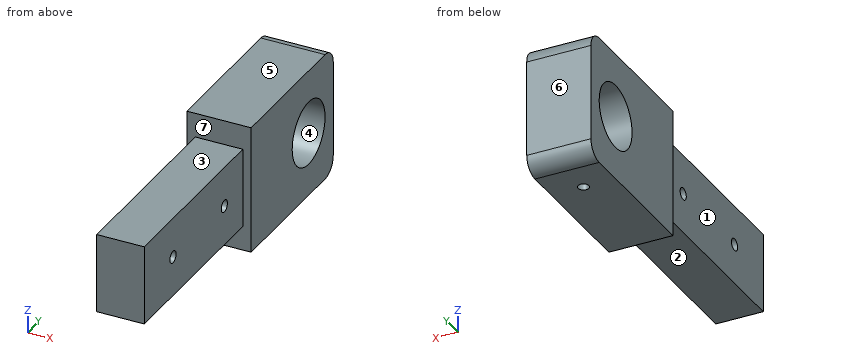
```python
from build123d import *

# Parameters (mm, degrees)
SKETCH2_W               = 20.828
SKETCH2_H               = 33.528
BOSS_EXTRUDE1_DEPTH     = 76.2
SKETCH3_W               = 25.4
SKETCH3_H               = 50.8
BOSS_EXTRUDE2_DEPTH     = 63.5
FILLET1_R               = 6.35
SKETCH4_R               = 12.7
CUT_EXTRUDE1_DEPTH      = 145.244271983
CUT_EXTRUDE2_REACH      = 151.191
CUT_EXTRUDE2_END_RADIUS = 12.7
SKETCH5_R               = 2.15265
SKETCH6_W               = 20.828
SKETCH6_H               = 33.528
CUT_EXTRUDE3_DEPTH      = 76.2
SKETCH7_R               = 2.38125
CUT_EXTRUDE4_DEPTH      = 78.74


with BuildPart() as part:
    # Sketch2 → Boss-Extrude1 (new body)
    with BuildSketch(Plane(origin=(0, 0, 0), x_dir=(1, 0, 0), z_dir=(0, 1, 0))):
        Rectangle(SKETCH2_W, SKETCH2_H)
    extrude(amount=BOSS_EXTRUDE1_DEPTH)

    # Sketch3 → Boss-Extrude2 (add)
    with BuildSketch(Plane(origin=(0, 76.2, 0), x_dir=(1, 0, 0), z_dir=(0, 1, 0))):
        Rectangle(SKETCH3_W, SKETCH3_H)
    extrude(amount=BOSS_EXTRUDE2_DEPTH)

    # Fillet1
    fillet1_edges = [part.edges().sort_by_distance(p)[0] for p in [
        (0, 139.7, -25.4),
        (0, 139.7, 25.4),
    ]]
    fillet(fillet1_edges, radius=FILLET1_R)

    # Sketch4 → Cut-Extrude1 (cut, through all)
    with BuildSketch(Plane(origin=(12.7, 0, 0), x_dir=(0, 0, -1), z_dir=(1, 0, 0))):
        with Locations((0, 120.65)):
            Circle(SKETCH4_R)
    extrude(amount=-CUT_EXTRUDE1_DEPTH, mode=Mode.SUBTRACT)

    # Cut-Extrude2: up to this cylinder (the profile starts outside it)
    cut_extrude2_end = Plane(origin=(0, 120.65, 0), z_dir=(1, 0, 0)) * Cylinder(CUT_EXTRUDE2_END_RADIUS, 328.782, mode=Mode.PRIVATE)
    # Sketch5 → Cut-Extrude2 (cut, up to the surface)
    with BuildSketch(Plane(origin=(0, 0, -25.4), x_dir=(-1, 0, 0), z_dir=(0, 0, -1)), mode=Mode.PRIVATE) as cut_extrude2_sk1:
        with Locations((0, 120.65)):
            Circle(SKETCH5_R)
    cut_extrude2_tool1 = extrude(cut_extrude2_sk1.sketch, amount=-CUT_EXTRUDE2_REACH, mode=Mode.PRIVATE) - cut_extrude2_end
    add(cut_extrude2_tool1.solids().sort_by_distance((0, 120.65, -25.4))[0], mode=Mode.SUBTRACT)

    # Sketch6 → Cut-Extrude3 (cut)
    with BuildSketch(Plane.XZ):
        Rectangle(SKETCH6_W, SKETCH6_H)
        Polygon((-9.398, -15.748), (-9.398, 15.748), (0, 15.748), (9.398, 15.748), (9.398, -15.748), align=None, mode=Mode.SUBTRACT)
    extrude(amount=-CUT_EXTRUDE3_DEPTH, mode=Mode.SUBTRACT)

    # Sketch7 → Cut-Extrude4 (cut)
    with BuildSketch(Plane(origin=(9.398, 0, 0), x_dir=(0, 0, -1), z_dir=(1, 0, 0))):
        with Locations((0, 61.9125)):
            Circle(SKETCH7_R)
        with Locations((0, 22.225)):
            Circle(SKETCH7_R)
    extrude(amount=-CUT_EXTRUDE4_DEPTH, mode=Mode.SUBTRACT)


solid = part.part
```
Source: CAD feature listing. Evaluate the final solid. Frame: model axes, mm. Face numbers are marked on the shaded views. A direction names the side the tool comes from. Round coordinates to 2 decimals unless told otherwise and drop trailing zeros. Write each loop counter-clockwise with the first axis right and the second up, starting at its lowest first coordinate (ties: lowest second). Pieces come first, ordered by that corner, then holes. Notation, with made-up numbers: M -38.5,-40 L -10.5,-40 A13 cw -10.5,-22 Z; hole C 81.25,-12 d2. An arc over 180 degrees is marked long. Use CSV: the item, a comma, the result in double quotes. Start each with the question number.
Q1. Cut plane D-D on z = -20.5. Output: boundary loops of the cut face in (x, y).
Q2. Access query for the marked faces 1, 2 and 3. Directions: +Z, -Z, +X, -X, +Y, -Y. A direction counts if a zero-diameter tool reaches every point of the face in a straight line with its end or side. Return the directions, or none.
Q3. Cut plane A-A on z = 0. Output: boundary loops of the cut face in (x, y), plus the area to 3 significant figures.
Q4. First-contact query: P1, Ø10, axis at x = 1, y = 20, coming from the +Z side; P2, Ø6, axis at y = 64.5, z = 1.5, coming from the -X side; P3, Ø15, axis at x = -3.5, y = 28, coming from the -Z side. Flat tips, straight axial feed; report the tip coordinate or a pass-through.
Q5. Line query: line 1 (Y direction, x = 3.75, z = 0); line 2 (Y direction, x = -0.25, z = 16); line 3 (Y direction, x = -8.75, z = -1). Output: solid intervals per line, ascending. Write a range as from..to.
Q6. Pull-direction query (Y, two-part tool) for the marked faces 4, 5, 6 and 7; classes: +Y half, -Y half, draft (parallel to the pull), parting line (faces both ways), or undercut.
Q7. Cut plane B-B on y = 120.65. Output: boundary loops of the cut face in (x, z).
Q8. Cut plane C-C on x = 4. Count the separate pieces of the cut face and the enclosed holes in it, plus the area to 3 significant figures.
Results found:
1,outline,"M -12.7,76.2 L 12.7,76.2 L 12.7,139.53 L -12.7,139.53 Z; hole C 0,120.65 d4.31"
2,face 1,"+Z, -Z, -X, -Y"
2,face 2,"-Z, +X, -X, -Y"
2,face 3,"+Z, +X, -X, -Y"
3,outline,"M -12.7,76.2 L -9.4,76.2 L -9.4,64.29 L 9.4,64.29 L 9.4,76.2 L 12.7,76.2 L 12.7,107.95 L -12.7,107.95 Z; M -12.7,133.35 L 12.7,133.35 L 12.7,139.7 L -12.7,139.7 Z; M -9.4,0 L 9.4,0 L 9.4,19.84 L -9.4,19.84 Z; M -9.4,24.61 L 9.4,24.61 L 9.4,59.53 L -9.4,59.53 Z"
3,area,"2,220 mm^2"
4,P1,"z = 15.75"
4,P2,"x = -9.4"
4,P3,"z = -15.75"
5,line 1,"0..19.84, 24.61..59.53, 64.29..107.95, 133.35..139.7"
5,line 2,"76.2..139.7"
5,line 3,"0..20.06, 24.39..59.75, 64.07..107.99, 133.31..139.7"
6,face 4,"undercut"
6,face 5,"draft"
6,face 6,"+Y half"
6,face 7,"-Y half"
7,outline,"M -12.7,-25.4 L -2.15,-25.4 L -2.15,-12.7 L -12.7,-12.7 Z; M -12.7,12.7 L 12.7,12.7 L 12.7,25.4 L -12.7,25.4 Z; M 2.15,-25.4 L 12.7,-25.4 L 12.7,-12.7 L 2.15,-12.7 Z"
8,separate pieces,"1"
8,enclosed holes,"3"
8,area,"5,070 mm^2"
